Work out the finished part from the listing and answer in its coordinate system (mm). Face numbers are marked on the shaded views. A direction names the side the tool comes from. Coordinates: 2 decimals unless noted, no trailing zeros. Use a Markdown table: item, result.
from build123d import *

# Parameters (mm, degrees)
F0_R          = 6.35
F1_DEPTH      = 1.5875
F2_R          = 9.525
F2_R_2        = 6.35
F3_DEPTH      = 6.35
F4_R          = 12.065
F4_R_2        = 9.525
F5_DEPTH      = 2.032
F6_R          = 12.065
F6_R_2        = 6.35
F7_DEPTH      = 2.032
F9_DEPTH      = 6.35
F10_R         = 1.2005117183
F11_DEPTH     = 12.7
F12_T1_DEPTH  = 3.6932202738
F12_T6_ANGLE  = 313.32464119
F12_S7_R      = 1.2005117183
F12_T8_DEPTH  = 18
F12_T12_DEPTH = 2.8797396175
F12_S13_R     = 1.2005117183
F12_T14_DEPTH = 3
F12_T18_ANGLE = 313.32464119
F12_S19_R     = 1.2005117183
F12_T20_DEPTH = 18


# Not quite as in the source:
# - a fillet or chamfer that OpenCascade refuses, or shapes differently, is made with other operations: its cross-section is extruded or revolved along the edge and cut away or added


with BuildPart() as f1:
    # F0 (on Top) → F1 (new body)
    with BuildSketch(Plane.XY):
        Circle(F0_R)
        with BuildLine():
            ThreePointArc((1.4859, -1.9812), (0, -2.4765), (-1.4859, -1.9812))
            Line((-1.4859, -1.9812), (-1.4859, 1.9812))
            ThreePointArc((-1.4859, 1.9812), (0, 2.4765), (1.4859, 1.9812))
            Line((1.4859, 1.9812), (1.4859, -1.9812))
        make_face(mode=Mode.SUBTRACT)
    extrude(amount=-F1_DEPTH)

    # F2 (on face) → F3 (join)
    with BuildSketch(Plane(origin=(0, 0, -1.5875), x_dir=(1, 0, 0), z_dir=(0, 0, -1))):
        Circle(F2_R)
        Circle(F2_R_2, mode=Mode.SUBTRACT)
        Circle(F2_R_2)
        with BuildLine():
            ThreePointArc((-1.4859, 1.9812), (0, 2.4765), (1.4859, 1.9812))
            Line((1.4859, 1.9812), (1.4859, -1.9812))
            ThreePointArc((1.4859, -1.9812), (0, -2.4765), (-1.4859, -1.9812))
            Line((-1.4859, -1.9812), (-1.4859, 1.9812))
        make_face(mode=Mode.SUBTRACT)
    extrude(amount=F3_DEPTH)

    # F4 (on face) → F5 (join)
    with BuildSketch(Plane.XY.offset(-1.5875)):
        Circle(F4_R)
        Circle(F4_R_2, mode=Mode.SUBTRACT)
    extrude(amount=-F5_DEPTH)

    # F6 (on face) → F7 (join)
    with BuildSketch(Plane(origin=(0, 0, -7.9375), x_dir=(1, 0, 0), z_dir=(0, 0, -1))):
        Circle(F6_R)
        Circle(F6_R_2, mode=Mode.SUBTRACT)
    extrude(amount=-F7_DEPTH)

    # F8 (on face) → F9 (join)
    with BuildSketch(Plane.XY.offset(-1.5875)):
        with BuildLine():
            ThreePointArc((7.7828940639, 9.2190446897), (10.1726283334, 6.4870530898), (11.6416666667, 3.1679365875))
            Line((11.6416666667, 3.1679365875), (14.2287037037, 7.0398590833))
            ThreePointArc((14.2287037037, 7.0398590833), (13.6199100402, 8.1555916706), (12.9238090364, 9.2190446897))
            Line((12.9238090364, 9.2190446897), (7.7828940639, 9.2190446897))
        make_face()
        with BuildLine():
            ThreePointArc((2.3947525988, 9.2190446897), (7.534442365, 5.8273324299), (9.525, 0))
            Line((9.525, 0), (11.6416666667, 3.1679365875))
            ThreePointArc((11.6416666667, 3.1679365875), (10.1726283334, 6.4870530898), (7.7828940639, 9.2190446897))
            Line((7.7828940639, 9.2190446897), (2.3947525988, 9.2190446897))
        make_face()
    extrude(amount=-F9_DEPTH)

    # F10 (on face) → F11 (cut)
    with BuildSketch(Plane(origin=(6.5851851852, -4.399911927, 0), x_dir=(0.5555555556, 0.8314794193, 0), z_dir=(0.8314794193, -0.5555555556, 0))):
        with Locations((10.2023333333, -4.7625)):
            Circle(F10_R)
    extrude(amount=-F11_DEPTH, mode=Mode.SUBTRACT)

    # F12: fillet of radius 0.9525 on 4 edges, made by hand

    # F12_s2 → F12_t1 (join)
    with BuildSketch(Plane.XY.offset(-6.6091101369)):
        with BuildLine():
            ThreePointArc((9.6813578082, 0.2340149392), (9.5658390102, -0.0058514421), (9.5212199592, -0.2683197522))
            ThreePointArc((9.5212199592, -0.2683197522), (9.5240549429, -0.1341731886), (9.525, 0))
            Line((9.525, 0), (9.6813578082, 0.2340149392))
        make_face()
    extrude(amount=F12_T1_DEPTH)


with BuildPart() as f12_tool4:
    # F12_s5 → F12_t6 (revolve)
    with BuildSketch(Plane(origin=(0, 0, 0), x_dir=(0, 0, 1), z_dir=(0.8751013478, -0.4839396977, 0))):
        with BuildLine():
            ThreePointArc((-3.6195, -10.4775), (-3.8984807909, -9.8039807909), (-4.572, -9.525))
            Line((-4.572, -9.525), (-3.6195, -9.525))
            Line((-3.6195, -9.525), (-3.6195, -10.4775))
        make_face()
    revolve(axis=Axis((0, 0, -3.6195), (0, 0, 1)), revolution_arc=F12_T6_ANGLE)

    # F12_s7 → F12_t8 (cut, symmetric)
    with BuildSketch(Plane(origin=(0, 0, 0), x_dir=(0, 0, 1), z_dir=(0.8314794193, -0.5555555556, 0))):
        with Locations((-4.7625, -10.2023333333)):
            Circle(F12_S7_R)
    extrude(amount=F12_T8_DEPTH, both=True, mode=Mode.SUBTRACT)


with BuildPart() as f1_1:
    add(f1.part)

    # F12_t3: union F12_tool4
    add(f12_tool4.part)


with BuildPart() as f12_tool10:
    # F12_s11 → F12_t12 (new body)
    with BuildSketch(Plane.XY.offset(-3.3226301913)):
        with BuildLine():
            ThreePointArc((2.2850004748, 9.2468588088), (2.398407194, 9.2260237879), (2.5135005223, 9.2190446897))
            Line((2.5135005223, 9.2190446897), (2.3947525988, 9.2190446897))
            ThreePointArc((2.3947525988, 9.2190446897), (2.3399178648, 9.2331148258), (2.2850004748, 9.2468588088))
        make_face()
    extrude(amount=-F12_T12_DEPTH)

    # F12_s13 → F12_t14 (cut, symmetric)
    with BuildSketch(Plane(origin=(-2.5775861998, 1.7222222222, 0), x_dir=(0, 0, 1), z_dir=(0.8314794193, -0.5555555556, 0))):
        with Locations((-4.7625, -10.2023333333)):
            Circle(F12_S13_R)
    extrude(amount=F12_T14_DEPTH, both=True, mode=Mode.SUBTRACT)


with BuildPart() as f1_2:
    add(f1_1.part)

    # F12_t9: union F12_tool10
    add(f12_tool10.part)


with BuildPart() as f12_tool16:
    # F12_s17 → F12_t18 (revolve)
    with BuildSketch(Plane(origin=(0, 0, 0), x_dir=(0, 0, 1), z_dir=(0.8751013478, -0.4839396977, 0))):
        with BuildLine():
            ThreePointArc((-5.9055, -10.4775), (-5.6265192091, -9.8039807909), (-4.953, -9.525))
            Line((-4.953, -9.525), (-5.9055, -9.525))
            Line((-5.9055, -9.525), (-5.9055, -10.4775))
        make_face()
    revolve(axis=Axis((0, 0, -5.9055), (0, 0, 1)), revolution_arc=F12_T18_ANGLE)

    # F12_s19 → F12_t20 (cut, symmetric)
    with BuildSketch(Plane(origin=(0, 0, 0), x_dir=(0, 0, 1), z_dir=(0.8314794193, -0.5555555556, 0))):
        with Locations((-4.7625, -10.2023333333)):
            Circle(F12_S19_R)
    extrude(amount=F12_T20_DEPTH, both=True, mode=Mode.SUBTRACT)


with BuildPart() as f1_3:
    add(f1_2.part)

    # F12_t15: union F12_tool16
    add(f12_tool16.part)


solid = f1_3.part
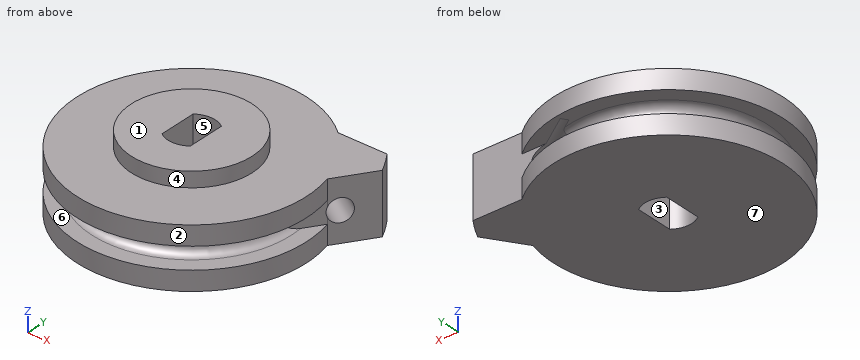
(1) Which of the six approach directions +Z, -Z, +X, -X, +Y, -Y give full straight-line access (tool end or side, diameter ignored) to the marked faces 4, 5, 6 and 7?
Conclusion:
| item | result |
|---|---|
| face 4 | +Z |
| face 5 | +Z, -Z |
| face 6 | none |
| face 7 | -Z, +X, -X, +Y, -Y |
(2) Determine the mould class of the marked faces 1, 2 and 3 for opening direction X: pulls with the +X half, pulls with the -X half, needs draft (parallel to the pull), parting line crosses it, or undercut.
Conclusion:
| item | result |
|---|---|
| face 1 | needs draft |
| face 2 | parting line crosses it |
| face 3 | undercut |
(3) Straight lines are drawn through the part: L1, parallel to Z at x = -9.5, y = 7; L2, parallel to X at y = 0, z = -7 (3 decimals); L3, parallel to Z at x = 9, y = 2.5. For each, find the intervals that lie inside material, in ascending order.
Conclusion:
| item | result |
|---|---|
| L1 | -7.94 to -5.91, -3.62 to -1.59 |
| L2 | -12.065 to -1.486, 1.486 to 12.065 |
| L3 | -7.94 to -1.59 |
(4) Given P1, Ø3, axis at x = -1.5, z = -4.5, coming from the -Y side; P2, Ø2, axis at x = -4.5, z = -5, coming from the -Y side; P3, Ø3, axis at y = 5.5, z = -4, coming from the -X side, each flat-ended and moving along its own axis, determine where each tip first touches the part or whether it passes through.
Conclusion:
| item | result |
|---|---|
| P1 | y = -12.06 |
| P2 | y = -11.36 |
| P3 | x = -11.37 |
